```python
from build123d import *

# Parameters (mm, degrees)
SKETCH1_W           = 55
SKETCH1_H           = 93
BOSS_EXTRUDE1_DEPTH = 3
CUT_EXTRUDE2_DEPTH  = 3


with BuildPart() as part:
    # Sketch1 → Boss-Extrude1 (new body)
    with BuildSketch(Plane.XY):
        Rectangle(SKETCH1_W, SKETCH1_H)
    extrude(amount=BOSS_EXTRUDE1_DEPTH)

    # Sketch2 → Cut-Extrude2 (cut)
    with BuildSketch(Plane.XY.offset(3)):
        Polygon((-27.5, 46.5), (-19.5, 46.5), (-15, 46.5), (-15, 43.5), (-24.5, 43.5), (-24.5, 10), (-27.5, 10), align=None)
        Polygon((-27.5, -46.5), (-27.5, -10), (-24.5, -10), (-24.5, -43.5), (-15, -43.5), (-15, -46.5), (-19.5, -46.5), align=None)
        Polygon((27.5, -46.5), (19.5, -46.5), (15, -46.5), (15, -43.5), (24.5, -43.5), (24.5, -10), (27.5, -10), align=None)
        Polygon((27.5, 46.5), (27.5, 10), (24.5, 10), (24.5, 43.5), (15, 43.5), (15, 46.5), (19.5, 46.5), align=None)
    extrude(amount=-CUT_EXTRUDE2_DEPTH, mode=Mode.SUBTRACT)


solid = part.part
```
Model file for the job. Use its own axes, mm. A direction names the side the tool comes from. Coordinates: 2 decimals unless noted, no trailing zeros. Order: outer loops, then holes, each group sorted by start corner. A loop starts at its lowest first (then second) coordinate and runs counter-clockwise, first axis right, second up. Notation, with made-up numbers: (45, 79.25) - (83, 79.25) arc R28 cw to (83, 116.25) - close; hole circle Ø11 at (-37.75, -2). An arc over 180 degrees is marked (long way). Return JSON: item names as keys, results as strings. Group by question number.
1) Probe line 1 (X direction, y = -36, z = 2); line 2 (Y direction, x = 18.5, z = 0.35). List the from-to ranges inside material, lowest first. Write a range as from..to.
2) Tool access for faces 1 (the flat face through (-15, 45, 2)), 2 (the flat face through (-15, -45, 2)), 3 (the flat face through (24.5, -27, 2)): list every direction of +Z, -Z, +X, -X, +Y, -Y with a clear straight run to the whole face (end or side of a thin tool).
3) Flat gauge pins, fed straight in: P1, Ø0.9, axis at y = -45, z = 1.5, coming from the +X side; P2, Ø1.5, axis at y = -32.5, z = 1.5, coming from the -X side; P3, Ø1, axis at x = -21, z = 1, coming from the -Y side. Where does each tip first touch, or does it go through?
4) Saw through at B-B, the plane x = -20. Write the cut outline in (y, z), plus the area to 3 significant figures.
5) Saw through at C-C, the plane y = -31. Write the cut outline in (x, z).
6) Saw through at A-A, the plane z = 2.55. Write the cut outline in (x, y), plus the area to 3 significant figures.
Values found:
{
 "1": {"line 1": "x = -24.5..24.5", "line 2": "y = -43.5..43.5"},
 "2": {"face 1": "+Z, -Z, -X, +Y", "face 2": "+Z, -Z, -X, -Y", "face 3": "+Z, -Z, +X, -Y"},
 "3": {"P1": "stops at x = 15", "P2": "stops at x = -24.5", "P3": "stops at y = -43.5"},
 "4": {"outline": "(-43.5, 0) - (43.5, 0) - (43.5, 3) - (-43.5, 3) - close", "area": "261 mm²"},
 "5": {"outline": "(-24.5, 0) - (24.5, 0) - (24.5, 3) - (-24.5, 3) - close"},
 "6": {"outline": "(-27.5, -10) - (-24.5, -10) - (-24.5, -43.5) - (-15, -43.5) - (-15, -46.5) - (15, -46.5) - (15, -43.5) - (24.5, -43.5) - (24.5, -10) - (27.5, -10) - (27.5, 10) - (24.5, 10) - (24.5, 43.5) - (15, 43.5) - (15, 46.5) - (-15, 46.5) - (-15, 43.5) - (-24.5, 43.5) - (-24.5, 10) - (-27.5, 10) - close", "area": "4,560 mm²"}
}
